Design review of the part built by this model. Coordinates are the model's own, in mm. Round coordinates to 2 decimals unless told otherwise and drop trailing zeros. Loops run counter-clockwise (first coordinate to the right, second up) from the corner with the lowest first, then second, coordinate; pieces in that order, holes last. Notation, with made-up numbers: (47, -12.5) - (101, -12.5) arc R25 ccw to (101, 15.5) - close; hole circle Ø3 at (13, 32.25). An arc over 180 degrees is marked (long way). Answer as CSV lines item,"result". Start each with the question number.
(1) Wall thickness on L1, parallel to X at y = -3.75, z = -2; L2, parallel to Z at x = 45, y = -4.75; L3, parallel to Z at x = 0, y = -4.75: over which ranges is each line inside the solid? List them lowest first.
(2) Mouldability with a two-part tool opening along Y and no side actions: class faces 1 (the flat face through (15, -15, 0)), 2 (the cylindrical face through (-1.5, -7.4, 11.4)), 3 (the flat face through (79.735, -7.423, 3.451)) as released by +Y, released by -Y, zero draft, split by the parting line, or undercut.
(3) Consider section D-D (x = -34). Give the boundary of the cut face in (y, z), and give its area (3 significant figures).
(4) Consider section A-A (z = 0). Give the boundary of the cut face in (x, y).
(5) Consider section B-B (x = 60). Give the boundary of the cut face in (y, z), and give its area (3 significant figures).
(6) Consider section C-C (x = 5). Give the boundary of the cut face in (y, z).
(7) For P1, Ø8, axis at y = -5, z = 9, coming from the -X side; P2, Ø6, axis at x = 41.5, y = -9, coming from the +Z side; P3, Ø8, axis at x = -43.5, y = -3, coming from the +Z side, all flat-tipped, find the tip position at first contact; note any pin that passes through.
from build123d import *

# Parameters (mm, degrees)
F0_R     = 11.5
F1_DEPTH = 15
F3_D     = 5.5
F4_D     = 13.2
F5_R     = 5.5
F6_DEPTH = 4.2


with BuildPart() as f1:
    # F0 (on Front) → F1 (new body)
    with BuildSketch(Plane.XZ):
        with BuildLine():
            Line((71.7835429594, 10.8070662041), (0, 20))
            Line((0, 20), (-51.8216221637, 12.3665554094))
            ThreePointArc((-51.8216221637, 12.3665554094), (-62.5, 0), (-51.8216221637, -12.3665554094))
            Line((-51.8216221637, -12.3665554094), (0, -20))
            Line((0, -20), (90.6974930025, -3.9387185113))
            ThreePointArc((90.6974930025, -3.9387185113), (94, 0), (90.6974930025, 3.9387185113))
            Line((90.6974930025, 3.9387185113), (71.7835429594, 10.8070662041))
        make_face()
        Circle(F0_R, mode=Mode.SUBTRACT)
    extrude(amount=F1_DEPTH)

    # F3 (through all)
    with Locations(Plane(origin=(0, 0, 0), x_dir=(-1, 0, 0), z_dir=(0, 1, 0))):
        with Locations((-60, 0), (-45, 0)):
            Hole(F3_D / 2)

    # F4 (through all)
    with Locations(Plane(origin=(0, 0, 0), x_dir=(1, 0, 0), z_dir=(0, 1, 0))):
        with Locations((-50, 0)):
            Hole(F4_D / 2)

    # F5 (on face) → F6 (cut)
    with BuildSketch(Plane(origin=(11.8303595902, 0, 32.5782619474), x_dir=(0.9399441976, 0, -0.3413281491), z_dir=(0.3413281491, 0, 0.9399441976))):
        with Locations((73.8449777845, -7.5)):
            Circle(F5_R)
    extrude(amount=-F6_DEPTH, mode=Mode.SUBTRACT)


solid = f1.part
Determined:
1,L1,"x = -62.34 to -56.29, -43.71 to -11.32, 11.32 to 43.11, 46.89 to 58.11, 61.89 to 93.46"
1,L2,"z = -12.03 to -2.75, 2.75 to 14.24"
1,L3,"z = -20 to -11.5, 11.5 to 20"
2,face 1,"released by -Y"
2,face 2,"zero draft"
2,face 3,"undercut"
3,outline,"(-15, -14.99) - (0, -14.99) - (0, 14.99) - (-15, 14.99) - close"
3,area,"450 mm^2"
4,outline,"(-62.5, -15) - (-56.6, -15) - (-56.6, 0) - (-62.5, 0) - close; (-43.4, -15) - (-11.5, -15) - (-11.5, 0) - (-43.4, 0) - close; (11.5, -15) - (42.25, -15) - (42.25, 0) - (11.5, 0) - close; (47.75, -15) - (57.25, -15) - (57.25, 0) - (47.75, 0) - close; (62.75, -15) - (94, -15) - (94, 0) - (62.75, 0) - close"
5,outline,"(-15, -9.37) - (0, -9.37) - (0, -2.75) - (-15, -2.75) - close; (-15, 2.75) - (0, 2.75) - (0, 12.32) - (-15, 12.32) - close"
5,area,"243 mm^2"
6,outline,"(-15, -19.11) - (0, -19.11) - (0, -10.36) - (-15, -10.36) - close; (-15, 10.36) - (0, 10.36) - (0, 19.36) - (-15, 19.36) - close"
7,P1,"stops at x = -61.46"
7,P2,"stops at z = 15.07"
7,P3,"stops at z = 14.18"
